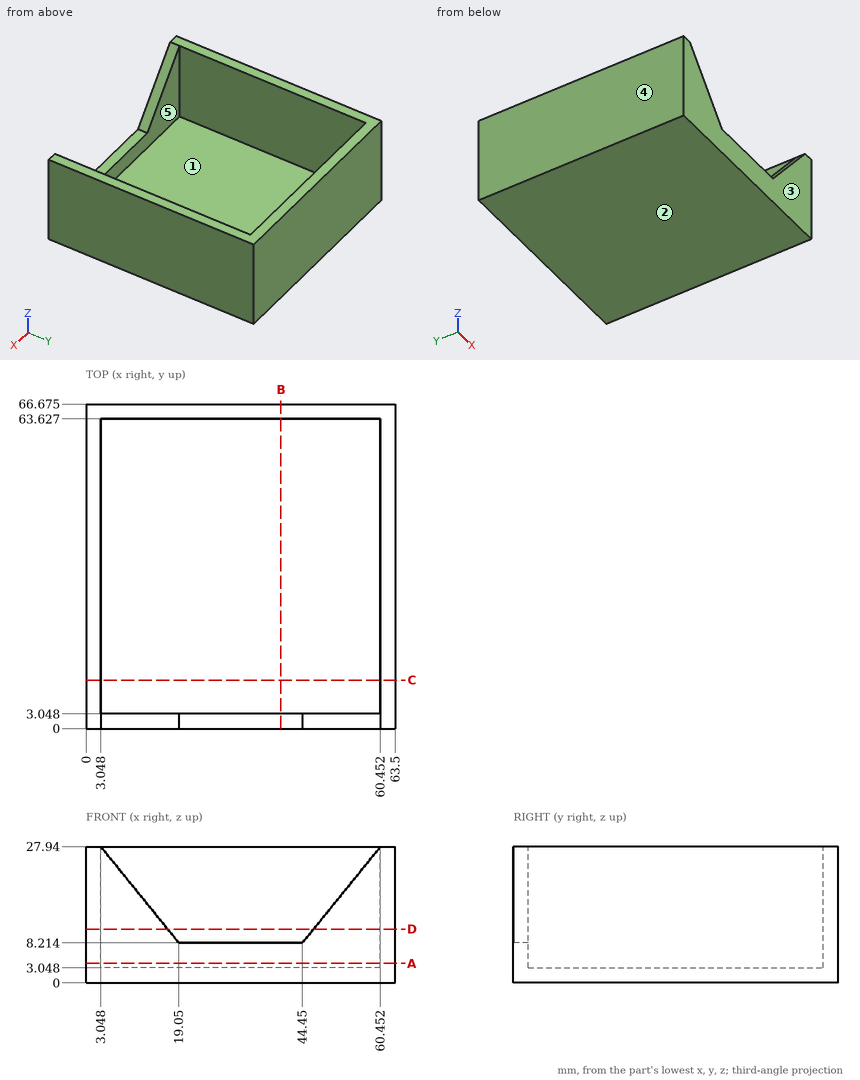
Can you work these out from the drawing? Everything is in mm from the part's minimum corner. A direction names the side the tool comes from. Coordinates: 2 decimals unless noted, no trailing zeros. Write each loop counter-clockwise with the first axis right and the second up, starting at its lowest first coordinate (ties: lowest second). Pieces come first, ordered by that corner, then holes. Notation, with made-up numbers: (77.5, -24.5) -> (110.5, -24.5) arc R24 cw to (110.5, -7.5) -> close; hole circle Ø4 at (48.25, -11.75). An arc over 180 degrees is marked (long way). Write each question's results on one line, items separated by ' | '. Start each with the question number.
Item 1: I'm going to push flat-ended pins straight in: P1, Ø2, axis at x = 48, y = 56, coming from the +Z side; P2, Ø0.9, axis at x = 28, y = 1, coming from the +Z side. Where does each tip first touch, or does it pass through?
Item 2: Please list where these lines run through material, in increasing order: probe 1 along Y at (x, z) = (6.5, 16.75) (1 decimal); probe 2 along X at (y, z) = (17, 5.5); probe 3 along X at (y, z) = (3, 17.5) (1 decimal).
Item 3: If we section it at B-B, the plane x = 40: Write out the boundary of the cut face in (y, z) (1 decimal), and give its area (3 significant figures).
Item 4: Thinking about a two-plate mould opening in Y: for the marked faces 3, 4 and 5, which applies, released by +Y, released by -Y, zero draft, split by the parting line, or undercut?
Item 5: If we section it at A-A, the plane z = 4: Write out the boundary of the cut face in (x, y) (1 decimal).
Item 6: On a 3-axis mill with a long thin cutter (end or side, diameter ignored), from which of +Z, -Z, +X, -X, +Y, -Y can I reach the whole of each face in a straight line? I mean the marked faces 1 and 2. Say none if no direction works.
Item 7: If we section it at D-D, the plane z = 11: Write out the boundary of the cut face in (x, y) (1 decimal).
Item 8: If we section it at C-C, the plane y = 10: Write out the boundary of the cut face in (x, z).
Answer block:
1) P1: z = 3.05 | P2: z = 8.21
2) probe 1: 0 to 3, 63.6 to 66.7 | probe 2: 0 to 3.05, 60.45 to 63.5 | probe 3: 0 to 11.5, 52 to 63.5
3) outline: (0, 0) -> (66.7, 0) -> (66.7, 27.9) -> (63.6, 27.9) -> (63.6, 3) -> (3, 3) -> (3, 8.2) -> (0, 8.2) -> close | area: 295 mm²
4) face 3: released by -Y | face 4: zero draft | face 5: undercut
5) outline: (0, 0) -> (63.5, 0) -> (63.5, 66.7) -> (0, 66.7) -> close; hole (3, 3) -> (60.5, 3) -> (60.5, 63.6) -> (3, 63.6) -> close
6) face 1: +Z | face 2: -Z, +X, -X, +Y, -Y
7) outline: (0, 0) -> (16.8, 0) -> (16.8, 3) -> (3, 3) -> (3, 63.6) -> (60.5, 63.6) -> (60.5, 3) -> (46.7, 3) -> (46.7, 0) -> (63.5, 0) -> (63.5, 66.7) -> (0, 66.7) -> close
8) outline: (0, 0) -> (63.5, 0) -> (63.5, 27.94) -> (60.45, 27.94) -> (60.45, 3.05) -> (3.05, 3.05) -> (3.05, 27.94) -> (0, 27.94) -> close
